Design review of the part built by this model. Coordinates are the model's own, in mm. Face numbers are marked on the shaded views. Give positions to 0.01 mm unless a question says otherwise; leave off trailing zeros. Loops run counter-clockwise (first coordinate to the right, second up) from the corner with the lowest first, then second, coordinate; pieces in that order, holes last. Notation, with made-up numbers: (53.5, 83.25) -> (91.5, 83.25) arc R19 ccw to (91.5, 97.25) -> close; hole circle Ø7 at (46.25, -28). An arc over 180 degrees is marked (long way). Use CSV: the item, a comma, the result in double quotes. Start each with the question number.
Item 1: Wall thickness on line 1 along X through (y, z) = (46, 0) (1 decimal); line 2 along X through (y, z) = (45.5, -2); line 3 along Y through (x, z) = (-4, -4.5): over which ranges is each line inside the solid? List them lowest first. Write a range as from..to.
Item 2: We need section D-D (y = 19). State the section outline as (x, z) points (1 decimal).
Item 3: The part is to be moulded in two halves that separate along X. For the marked faces 1, 2 and 3, say which applies: +X half, -X half, draft (parallel to the pull), parting line (faces both ways), or undercut.
Item 4: Clearance check with flat-ended pins moving along their axes: pin 1 (3 mm diameter, centred on x = -1, y = 14, fed in from -Z); pin 2 (6 mm diameter, centred on y = 30, z = -2, fed in from +X); pin 3 (3 mm diameter, centred on x = -0.5, z = 1, fed in from +Y). State where each tip first meets the part, or that it passes through.
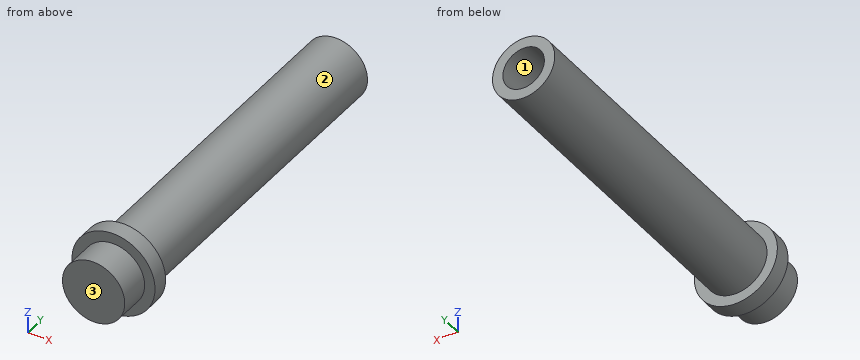
from build123d import *

# Parameters (mm, degrees)
SKETCH1_R           = 6.35
BOSS_EXTRUDE1_DEPTH = 2.54
SKETCH2_R           = 4.7625
BOSS_EXTRUDE2_DEPTH = 4.7625
BOSS_EXTRUDE3_START = 50.8
SKETCH3_R           = 4.7625
BOSS_EXTRUDE3_DEPTH = 50.8
SKETCH4_R           = 3.175
CUT_EXTRUDE1_DEPTH  = 25.4


with BuildPart() as part:
    # Sketch1 → Boss-Extrude1 (new body)
    with BuildSketch(Plane(origin=(0, 0, 0), x_dir=(1, 0, 0), z_dir=(0, 1, 0))):
        with Locations(Location((0, 0, 0), (0, 0, 270))):
            Circle(SKETCH1_R)
    extrude(amount=BOSS_EXTRUDE1_DEPTH)

    # Sketch2 → Boss-Extrude2 (add)
    with BuildSketch(Plane.XZ):
        with Locations(Location((0, 0, 0), (0, 0, 90))):
            Circle(SKETCH2_R)
    extrude(amount=BOSS_EXTRUDE2_DEPTH)

    # Sketch3 → Boss-Extrude3 (add)
    with BuildSketch(Plane(origin=(0, 2.54, 0), x_dir=(1, 0, 0), z_dir=(0, 1, 0)).offset(BOSS_EXTRUDE3_START)):
        with Locations(Location((0, 0, 0), (0, 0, 270))):
            Circle(SKETCH3_R)
    extrude(amount=-BOSS_EXTRUDE3_DEPTH)

    # Sketch4 → Cut-Extrude1 (cut)
    with BuildSketch(Plane(origin=(0, 53.34, 0), x_dir=(1, 0, 0), z_dir=(0, 1, 0))):
        with Locations(Location((0, 0, 0), (0, 0, 270))):
            Circle(SKETCH4_R)
    extrude(amount=-CUT_EXTRUDE1_DEPTH, mode=Mode.SUBTRACT)


solid = part.part
Results found:
1,line 1,"-4.8..-3.2, 3.2..4.8"
1,line 2,"-4.32..-2.47, 2.47..4.32"
1,line 3,"0..2.54"
2,outline,"circle Ø9.5 at (0, 0)"
3,face 1,"undercut"
3,face 2,"parting line"
3,face 3,"draft"
4,pin 1,"z = -4.76"
4,pin 2,"x = 4.76"
4,pin 3,"y = 27.94"
